Study the drawing (mm; zero at the part's minimum x, y, z) and answer. A direction names the side the tool comes from. Give positions to 0.01 mm unless a question says otherwise; leave off trailing zeros. Order: outer loops, then holes, each group sorted by start corner. A loop starts at its lowest first (then second) coordinate and runs counter-clockwise, first axis right, second up. Notation, with made-up numbers: (-1, 42.25) - (18, 42.25) arc R12 cw to (18, 49.25) - close; hole circle Ø1 at (-5, 15). An arc over 180 degrees is marked (long way). Put each result on its own line as item: value.
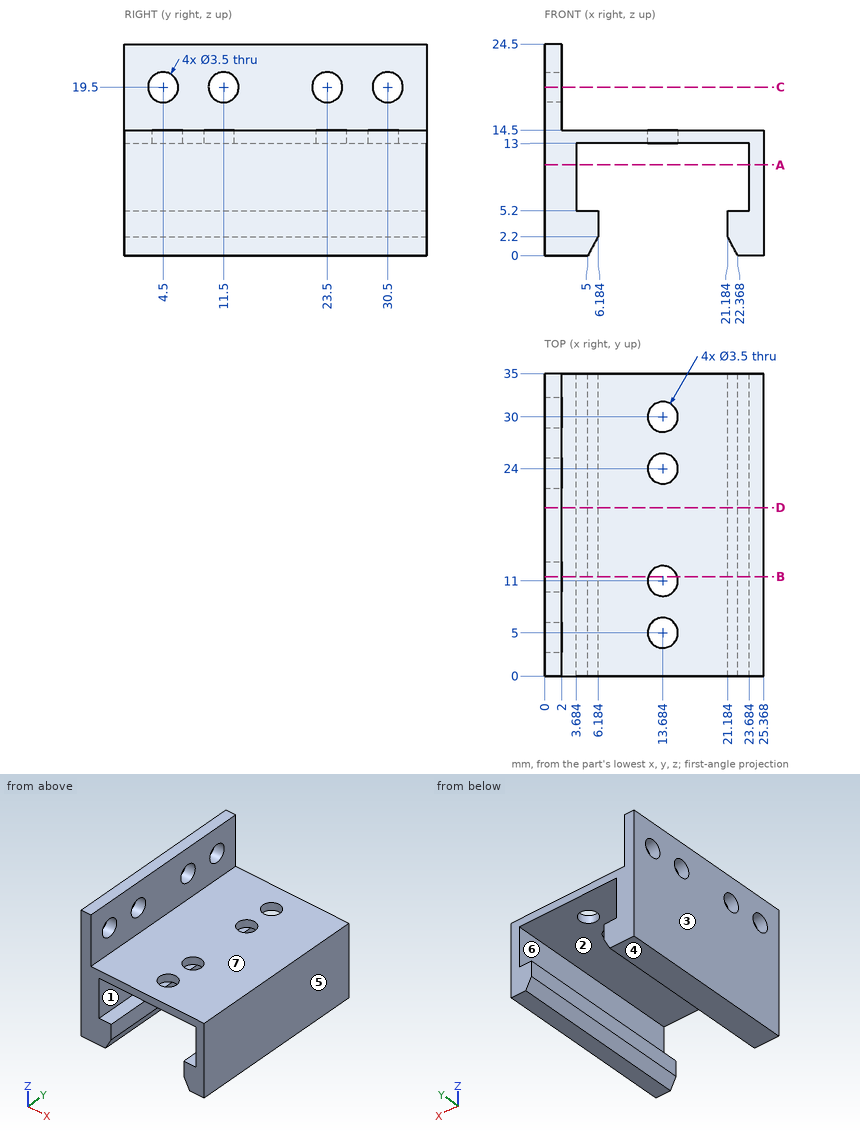
(1) Section C-C, the plane z = 19.5 is taken. Write down the section's boundary in (x, y), then the cut area to 3 significant figures.
Geometry check:
outline: (0, 0) - (2, 0) - (2, 2.75) - (0, 2.75) - close; (0, 6.25) - (2, 6.25) - (2, 9.75) - (0, 9.75) - close; (0, 13.25) - (2, 13.25) - (2, 21.75) - (0, 21.75) - close; (0, 25.25) - (2, 25.25) - (2, 28.75) - (0, 28.75) - close; (0, 32.25) - (2, 32.25) - (2, 35) - (0, 35) - close
area: 42.0 mm²
(2) Straight lines are drawn through the part: line 1 (Y direction, x = 1.35, z = 19.5); line 2 (X direction, y = 6.5, z = 9); line 3 (X direction, y = 5, z = 4). For each, find the intervals that lie inside material, in ascending order.
Geometry check:
line 1: y = 0 to 2.75, 6.25 to 9.75, 13.25 to 21.75, 25.25 to 28.75, 32.25 to 35
line 2: x = 0 to 3.68, 23.68 to 25.37
line 3: x = 0 to 6.18, 21.18 to 25.37
(3) A tool of negligible diameter and unlimited length cuts with its end or side. For the marked faces 5, 6 and 7, from which of +Z, -Z, +X, -X, +Y, -Y can it reach the whole face along a straight path? Write none if from no direction.
Geometry check:
face 5: +Z, -Z, +X, +Y, -Y
face 6: +Y, -Y
face 7: +Z, +X, +Y, -Y
(4) Section B-B, the plane y = 11.5 is taken. Write down the section's boundary in (x, z), then the cut area to 3 significant figures.
Geometry check:
outline: (0, 0) - (5, 0) - (6.18, 2.2) - (6.18, 5.2) - (3.68, 5.2) - (3.68, 13) - (12.01, 13) - (12.01, 14.5) - (2, 14.5) - (2, 17.75) - (0, 17.75) - close; (0, 21.25) - (2, 21.25) - (2, 24.5) - (0, 24.5) - close; (15.36, 13) - (23.68, 13) - (23.68, 5.2) - (21.18, 5.2) - (21.18, 2.2) - (22.37, 0) - (25.37, 0) - (25.37, 14.5) - (15.36, 14.5) - close
area: 139 mm²
(5) Section A-A, the plane z = 10.5 is taken. Write down the section's boundary in (x, y), then the cut area to 3 significant figures.
Geometry check:
outline: (0, 0) - (3.68, 0) - (3.68, 35) - (0, 35) - close; (23.68, 0) - (25.37, 0) - (25.37, 35) - (23.68, 35) - close
area: 188 mm²
(6) Section D-D, the plane y = 19.5 is taken. Write down the section's boundary in (x, z), then the cut area to 3 significant figures.
Geometry check:
outline: (0, 0) - (5, 0) - (6.18, 2.2) - (6.18, 5.2) - (3.68, 5.2) - (3.68, 13) - (23.68, 13) - (23.68, 5.2) - (21.18, 5.2) - (21.18, 2.2) - (22.37, 0) - (25.37, 0) - (25.37, 14.5) - (2, 14.5) - (2, 24.5) - (0, 24.5) - close
area: 151 mm²
(7) Determine the mould class of the marked faces 1, 2, 3 and 4 for opening direction X: pulls with the +X half, pulls with the -X half, needs draft (parallel to the pull), parting line crosses it, or undercut.
Geometry check:
face 1: undercut
face 2: undercut
face 3: pulls with the -X half
face 4: needs draft
(8) Given pin 1 (5.5 mm diameter, centred on y = 4.5, z = 19.5, fed in from +X); pin 2 (7 mm diameter, centred on x = 17.5, y = 25, fed in from +Z); pin 3 (3 mm diameter, centred on x = 18, z = 5, fed in from -Y); pin 4 (4.5 mm diameter, centred on x = 13.68, y = 30, fed in from -Z), each flat-ended and moving along its own axis, determine where each tip first touches the part or whether it passes through.
Geometry check:
pin 1: stops at x = 2
pin 2: stops at z = 14.5
pin 3: passes through
pin 4: stops at z = 13
